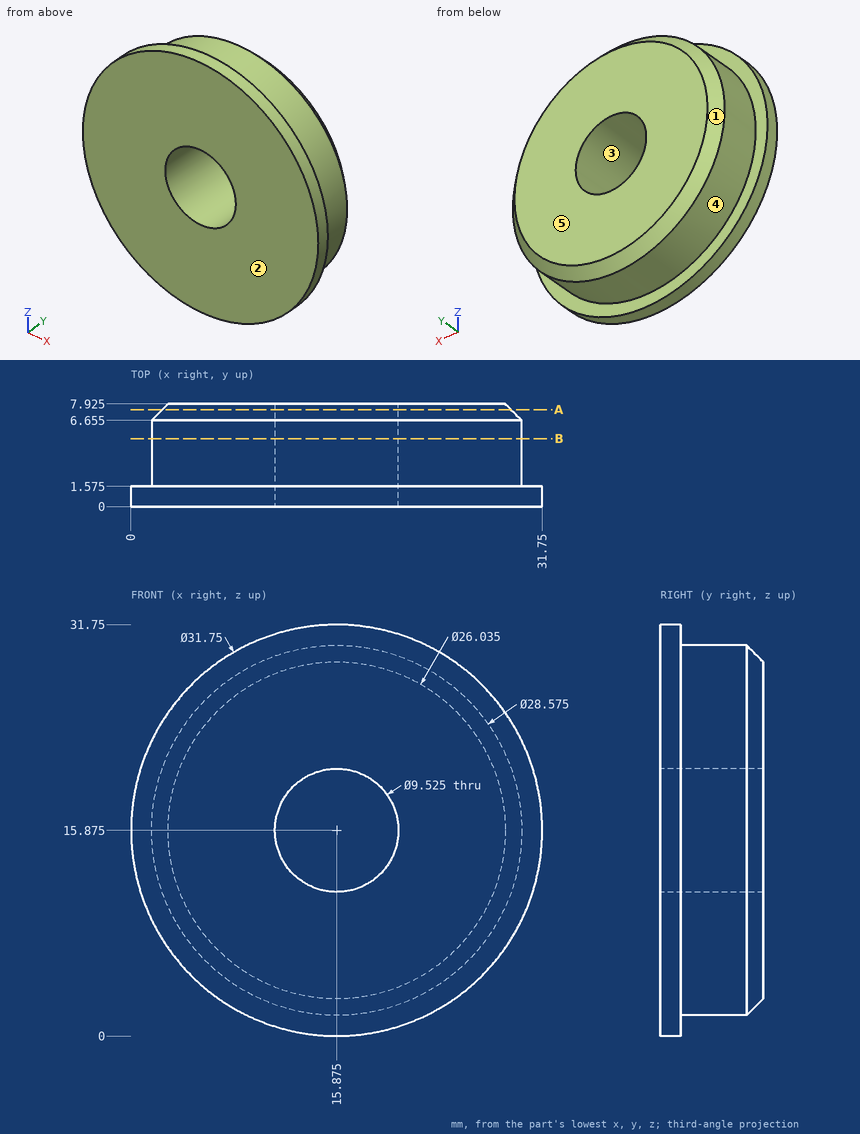
Drawing for the job (mm, zero at the part's lowest x, y, z). A direction names the side the tool comes from. Coordinates: 2 decimals unless noted, no trailing zeros. Order: outer loops, then holes, each group sorted by start corner. A loop starts at its lowest first (then second) coordinate and runs counter-clockwise, first axis right, second up.
Item 1: Two-plate mould, pull along Z, no slides. Class the marked faces 1, 2 and 3: +Z half, -Z half, draft (parallel to the pull), parting line (faces both ways), or undercut.
Check sheet entries:
face 1: parting line
face 2: draft
face 3: undercut
Item 2: 3-axis set-ups, long thin cutter, end or side, ignore diameter. For the marked faces 4 and 5: which of +Z, -Z, +X, -X, +Y, -Y reach the whole face in a straight line?
Check sheet entries:
face 4: +Y
face 5: +Z, -Z, +X, -X, +Y
Item 3: Pin check, flat tips, straight feed: pin 1 Ø1.5 at (y, z) = (7, 15) entering from +X; pin 2 Ø8.5 at (x, z) = (15.875, 15.875) entering from +Y; pin 3 Ø1.5 at (y, z) = (2, 20) entering from -X; pin 4 Ø1.5 at (y, z) = (7, 23.5) entering from -X. Stop position of each tip, or through.
Check sheet entries:
pin 1: stops at x = 30.16
pin 2: passes through
pin 3: stops at x = 0.39
pin 4: stops at x = 3.4
Item 4: Band-saw the part on A-A on y = 7.5. List the corners of the cut face in (x, z) (1 decimal), plus the area to 3 significant figures.
Check sheet entries:
outline: circle Ø26.9 at (15.9, 15.9); hole circle Ø9.5 at (15.9, 15.9)
area: 496 mm2
Item 5: Drill centre lines: L1, parallel to Z at x = 19, y = 5.75; L2, parallel to X at y = 1.5, z = 17.5. Where is each one in solid material? Low to high.
Check sheet entries:
L1: z = 1.93 to 12.28, 19.47 to 29.82
L2: x = 0.08 to 11.4, 20.35 to 31.67
Item 6: Band-saw the part on B-B on y = 5.25. List the corners of the cut face in (x, z) (1 decimal).
Check sheet entries:
outline: circle Ø28.6 at (15.9, 15.9); hole circle Ø9.5 at (15.9, 15.9)
